Source: CAD feature listing. Evaluate the final solid. Frame: model axes, mm. A direction names the side the tool comes from. Coordinates: 2 decimals unless noted, no trailing zeros. Loops run counter-clockwise (first coordinate to the right, second up) from the corner with the lowest first, then second, coordinate; pieces in that order, holes last.
Item 1: Pin query (flat end, axial travel): pin 1 Ø2.5 at (y, z) = (2.5, 2.5) entering from +X; pin 2 Ø1.5 at (y, z) = (3.5, 15) entering from -X. Return the tip coordinate at first contact, or that it passes through.
Item 2: Reachability of faces 4 (the flat face through (-14.288, 3, 13)), 5 (the flat face through (13, 46, 0)), 6 (the flat face through (0, 44.31, -11)) from +Z, -Z, +X, -X, +Y, -Y: full face, straight path, thin tool, end or side. Return the list, or none.
Item 3: Section query B-B, the plane x = 17.5. Return the cut outline in (y, z).
Item 4: Line query: probe 1 along Y at (x, z) = (8.5, 16); probe 2 along Z at (x, y) = (-19.5, 22); probe 3 along Y at (x, z) = (13.5, -12). Output: solid intervals per line, ascending.
Item 5: Section query C-C, the plane z = -16. Return the cut outline in (x, y).
Item 6: Pull-direction query (Y, two-part tool) for faces 1 (the flat face through (23.25, 27, 18)), 2 (the flat face through (-0.3, 47.4, 9.4)), 3 (the flat face through (5, 3, 9.028)); classes: +Y half, -Y half, draft (parallel to the pull), parting line (faces both ways), or undercut.
Item 7: Section query D-D, the plane y = 43. Return the cut outline in (x, z).
Autodesk Inventor part; units mm, degrees
ref_plane "YZ Plane" through (0, 0, 0) normal (1, 0, 0) x (0, 1, 0)
ref_plane "XZ Plane" through (0, 0, 0) normal (0, 1, 0) x (-1, 0, 0)
ref_plane "XY Plane" through (0, 0, 0) normal (0, 0, 1) x (1, 0, 0)
sketch "Sketch1" plane through (0, 0, 0) normal (0, 1, 0) x (-1, 0, 0)
  point P0 (0, 0)
sketch "Sketch2" plane through (0, 0, 0) normal (0, 1, 0) x (-1, 0, 0)
  line L0 (23.25, -20.5) -> (-23.25, -20.5)
  line L1 (-23.25, -20.5) -> (-23.25, 20.5)
  line L2 (-23.25, 20.5) -> (23.25, 20.5)
  line L3 (23.25, 20.5) -> (23.25, -20.5)
  line L4 (23.25, -20.5) -> (-23.25, 20.5) construction
  line L5 (-23.25, -20.5) -> (23.25, 20.5) construction
  point P0 (0, 0)
  dimension "d0" = 46.5
  dimension "d1" = 41
extrude "Extrusion1" add sketch "Sketch2" along normal blind 0.5
sketch "Sketch3" plane through (0, 0.5, 0) normal (0, 1, 0) x (1, 0, 0)
  line L0 (-13, -9) -> (13, -9)
  line L1 (13, -9) -> (13, 9)
  line L2 (13, 9) -> (-13, 9)
  line L3 (-13, 9) -> (-13, -9)
  line L4 (-13, -9) -> (13, 9) construction
  line L5 (13, -9) -> (-13, 9) construction
  point P0 (0, 0)
  dimension "d4" = 26
  dimension "d5" = 18
extrude "Extrusion2" cut sketch "Sketch3" against normal blind 25.4
sketch "Sketch4" plane through (0, 0.5, 0) normal (0, 1, 0) x (1, 0, 0)
  line L0 (-23.25, 20.5) -> (-23.25, -20.5)
  line L1 (23.25, -20.5) -> (23.25, 20.5)
  line L2 (-23.25, -20.5) -> (23.25, -20.5)
  line L3 (23.25, -20.5) -> (23.25, -17.4625)
  line L4 (23.25, -17.4625) -> (-23.25, -17.4625)
  line L5 (-23.25, -17.4625) -> (-23.25, -20.5)
  point P0 (0, 0)
extrude "Extrusion3" add sketch "Sketch4" along normal blind 46.9
sketch "Sketch5" plane through (0, 0.5, 0) normal (0, 1, 0) x (1, 0, 0)
  line L0 (-23.25, 20.5) -> (-23.25, -17.4625)
  line L1 (-23.25, 20.5) -> (23.25, 20.5)
  line L2 (23.25, 20.5) -> (23.25, 17.4625)
  line L3 (23.25, 17.4625) -> (-23.25, 17.4625)
  line L4 (-23.25, 17.4625) -> (-23.25, 20.5)
  point P0 (0, 0)
extrude "Extrusion4" add sketch "Sketch5" along normal blind 46.9
sketch "Sketch6" plane through (23.25, 0.5, 17.4625) normal (0, 0, -1) x (-1, 0, 0)
  point P0 (23.25, -0.5)
sketch "Sketch7" plane through (23.25, 0.5, 17.4625) normal (0, 0, -1) x (-1, 0, 0)
  point P0 (23.25, -0.5)
sketch "Sketch8" plane through (23.25, 0.5, 17.4625) normal (0, 0, -1) x (-1, 0, 0)
  line L0 (46.5, 0) -> (46.5, 46.9)
  line L1 (0, 0) -> (0, 46.9)
  line L2 (46.5, 46.9) -> (0, 46.9)
  line L3 (0, 46.9) -> (0, 43.8105)
  line L4 (0, 43.8105) -> (46.5, 43.8105)
  line L5 (46.5, 43.8105) -> (46.5, 46.9)
  point P0 (23.25, -0.5)
extrude "Extrusion5" add sketch "Sketch8" along normal blind 35
sketch "Sketch9" plane through (0, 47.4, 0) normal (0, 1, 0) x (1, 0, 0)
  line L0 (-13, -9) -> (-13, 9)
  line L1 (13, 9) -> (-13, 9)
  line L2 (-13, 9) -> (-13, -9)
  line L3 (-13, -9) -> (13, -9)
  line L4 (13, -9) -> (13, 9)
  line L5 (13, 9) -> (-13, -9) construction
  line L6 (-13, 9) -> (13, -9) construction
  point P0 (0, 0)
sketch "Sketch10" plane through (0, 0.5, 0) normal (0, 1, 0) x (1, 0, 0)
  point P0 (0, 0)
sketch "Sketch11" plane through (0, 0.5, 0) normal (0, 1, 0) x (1, 0, 0)
  line L0 (-23.25, -17.4625) -> (23.25, -17.4625)
  line L1 (-23.25, -17.4625) -> (-18.283, -17.4625)
  line L2 (-18.283, -17.4625) -> (-18.283, 17.4625)
  line L3 (-18.283, 17.4625) -> (-23.25, 17.4625)
  line L4 (-23.25, 17.4625) -> (-23.25, -17.4625)
  point P0 (0, 0)
extrude "Extrusion6" add sketch "Sketch11" along normal blind 2.9718
extrude "Extrusion7" cut sketch "Sketch9" against normal blind 4.9657
sketch "Sketch12" plane through (0, 0.5, 0) normal (0, 1, 0) x (1, 0, 0)
  point P0 (0, 0)
sketch "Sketch13" plane through (0, 0.5, 0) normal (0, 1, 0) x (1, 0, 0)
  line L0 (23.25, -17.4625) -> (23.25, 17.4625)
  line L1 (-14.2875, -17.4625) -> (23.25, -17.4625)
  line L2 (23.25, -17.4625) -> (23.25, -9.0284)
  line L3 (23.25, -9.0284) -> (-14.2875, -9.0284)
  line L4 (-14.2875, -9.0284) -> (-14.2875, -17.4625)
  point P0 (0, 0)
extrude "Extrusion8" add sketch "Sketch13" along normal blind 4.9657
properties part number "ChamberSurface"
Verdict:
1. pin 1: stops at x = -18.28
1. pin 2: stops at x = -23.25
2. face 4: none
2. face 5: +Y, -Y
2. face 6: +X, -X
3. outline: (0, -20.5) - (47.4, -20.5) - (47.4, 20.5) - (0, 20.5) - close; hole (0.5, -17.46) - (44.31, -17.46) - (44.31, 17.46) - (5.47, 17.46) - (5.47, 9.03) - (0.5, 9.03) - close
4. probe 1: y = 0 to 5.47, 44.31 to 47.4
4. probe 2: z = -20.5 to -17.46, 17.46 to 20.5
4. probe 3: y = 0 to 0.5, 44.31 to 47.4
5. outline: (-23.25, 0) - (23.25, 0) - (23.25, 0.5) - (-18.28, 0.5) - (-18.28, 3.47) - (-23.25, 3.47) - close; (-23.25, 44.31) - (23.25, 44.31) - (23.25, 47.4) - (-23.25, 47.4) - close
6. face 1: draft
6. face 2: +Y half
6. face 3: undercut
7. outline: (-23.25, -20.5) - (23.25, -20.5) - (23.25, -17.46) - (-23.25, -17.46) - close; (-23.25, 17.46) - (23.25, 17.46) - (23.25, 20.5) - (-23.25, 20.5) - close
